Input: part model. Units: mm. Frame: model coordinates. Face numbers are marked on the shaded views. Round coordinates to 2 decimals unless told otherwise and drop trailing zeros. Loops run counter-clockwise (first coordinate to the right, second up) from the corner with the lowest first, then second, coordinate; pieces in that order, holes last. Notation, with made-up numbers: (46, 71) - (62, 71) arc R12 cw to (62, 87) - close; hole circle Ø11 at (0.25, 33.25). An arc over 180 degrees is marked (long way). Write each question's results on one line, items separated by ' | '.
Autodesk Inventor part; units mm, degrees
ref_plane "YZ Plane" through (0, 0, 0) normal (1, 0, 0) x (0, 1, 0)
ref_plane "XZ Plane" through (0, 0, 0) normal (0, 1, 0) x (-1, 0, 0)
ref_plane "XY Plane" through (0, 0, 0) normal (0, 0, 1) x (1, 0, 0)
sketch "Sketch1" plane through (0, 0, 0) normal (0, 0, 1) x (1, 0, 0)
  circle A0 centre (0, 0) radius 10
  dimension "d0" = 20
extrude "Extrusion1" add sketch "Sketch1" along normal blind 2
sketch "Sketch2" plane through (0, 0, 2) normal (0, 0, 1) x (1, 0, 0)
  circle A0 centre (0, 0) radius 4.5
  dimension "d3" = 9
extrude "Extrusion2" add sketch "Sketch2" along normal blind 2.5
sketch "Sketch3" plane through (0, 0, 4.5) normal (0, 0, 1) x (1, 0, 0)
  circle A0 centre (0, 0) radius 1.5
  dimension "d6" = 3
extrude "Extrusion3" cut sketch "Sketch3" against normal through all
sketch "Sketch4" plane through (0, 0, 4.5) normal (0, 0, 1) x (1, 0, 0)
  circle A0 centre (0, 0) radius 3.025
  dimension "d9" = 6.05
extrude "Extrusion4" cut sketch "Sketch4" against normal blind 2.5
sketch "Sketch5" plane through (0, 0, 2) normal (0, 0, 1) x (1, 0, 0)
  line L0 (0, 0) -> (0, 7)
  circle A0 centre (0, 7) radius 1.5
  circle A1 centre (-7, 0) radius 1.5
  circle A2 centre (0, -7) radius 1.5
  circle A3 centre (7, 0) radius 1.5
  dimension "d12" = 7
  dimension "d13" = 3
  dimension "d16" = 360
extrude "Extrusion5" cut sketch "Sketch5" against normal through all
thread "Thread1"
thread "Thread2"
thread "Thread3"
thread "Thread4"
sketch "Sketch6" plane through (0, 0, 2) normal (0, 0, 1) x (1, 0, 0)
  circle A0 centre (0, 0) radius 3.025
extrude "Extrusion6" cut sketch "Sketch6" against normal blind 0.5
properties part number "servo_FT_SC_horn_1"
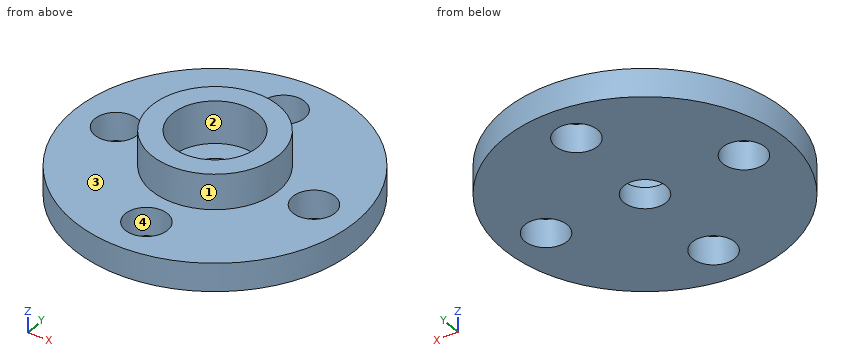
1. Section query C-C, the plane z = 0.4. Output: boundary loops of the cut face in (x, y).
Answer:
outline: circle Ø20 at (0, 0); hole circle Ø3 at (-7, 0); hole circle Ø3 at (0, -7); hole circle Ø3 at (0, 0); hole circle Ø3 at (0, 7); hole circle Ø3 at (7, 0)
2. Mould query, pull axis X, two halves, no side actions, for the marked faces 1, 2, 3 and 4. Classes: pulls with the +X half, pulls with the -X half, needs draft (parallel to the pull), parting line crosses it, or undercut.
Answer:
face 1: parting line crosses it | face 2: undercut | face 3: needs draft | face 4: undercut
3. Section query A-A, the plane y = 0. Output: boundary loops of the cut face in (x, z) (3 decimals), plus the area to 4 significant figures.
Answer:
outline: (-10, 0) - (-8.5, 0) - (-8.5, 2) - (-10, 2) - close; (-5.5, 0) - (-1.5, 0) - (-1.5, 1.5) - (-3.025, 1.5) - (-3.025, 4.5) - (-4.5, 4.5) - (-4.5, 2) - (-5.5, 2) - close; (1.5, 0) - (5.5, 0) - (5.5, 2) - (4.5, 2) - (4.5, 4.5) - (3.025, 4.5) - (3.025, 1.5) - (1.5, 1.5) - close; (8.5, 0) - (10, 0) - (10, 2) - (8.5, 2) - close | area: 27.85 mm^2
4. Contact query for flat-ended pins moving along their axis: pin 1 (4 mm diameter, centred on x = 0, y = 7, fed in from -Z); pin 2 (3.5 mm diameter, centred on x = 7, y = 0, fed in from +Z); pin 3 (1.8 mm diameter, centred on x = 1, y = -1, fed in from +Z); pin 4 (1 mm diameter, centred on x = 6.5, z = 1.5, fed in from +Y). Output: stop coordinate, or through.
Answer:
pin 1: z = 0 | pin 2: z = 2 | pin 3: z = 1.5 | pin 4: y = 8
5. Line query: line 1 (Y direction, x = 0, z = 1.1); line 2 (Z direction, x = 5.5, y = 6); line 3 (X direction, y = 0.75, z = 1.2). Output: solid intervals per line, ascending. Write a range as [from, to].
Answer:
line 1: [-10, -8.5], [-5.5, -1.5], [1.5, 5.5], [8.5, 10] | line 2: [0, 2] | line 3: [-9.97, -8.3], [-5.7, -1.3], [1.3, 5.7], [8.3, 9.97]
6. Section query D-D, the plane y = -7.5. Output: boundary loops of the cut face in (x, z).
Answer:
outline: (-6.61, 0) - (-1.41, 0) - (-1.41, 2) - (-6.61, 2) - close; (1.41, 0) - (6.61, 0) - (6.61, 2) - (1.41, 2) - close
